Part model, mm, in its own coordinate system. A direction names the side the tool comes from. Give positions to 0.01 mm unless a question says otherwise; leave off trailing zeros. Write each loop counter-clockwise with the first axis right and the second up, starting at its lowest first coordinate (ties: lowest second). Pieces come first, ordered by that corner, then holes. Notation, with made-up numbers: M 58,78.5 L 109,78.5 A28 ccw 109,116.5 Z; hole C 85.25,57.5 d10. An arc over 180 degrees is marked long. Use a Markdown table: item, result.
```python
from build123d import *

# Parameters (mm, degrees)
SKETCH1_R           = 20
BOSS_EXTRUDE1_DEPTH = 6
SKETCH2_R           = 2
SKETCH2_R_2         = 1.5
CUT_EXTRUDE1_DEPTH  = 6
SKETCH4_R           = 3
CUT_EXTRUDE2_DEPTH  = 3.1


with BuildPart() as part:
    # Sketch1 → Boss-Extrude1 (new body)
    with BuildSketch(Plane.XY):
        Circle(SKETCH1_R)
    extrude(amount=BOSS_EXTRUDE1_DEPTH)

    # Sketch2 → Cut-Extrude1 (cut)
    with BuildSketch(Plane(origin=(0, 0, 0), x_dir=(-1, 0, 0), z_dir=(0, 0, -1))):
        with Locations((0, 16)):
            Circle(SKETCH2_R)
        with Locations((11.313708499, 11.313708499)):
            Circle(SKETCH2_R)
        with Locations((16, 0)):
            Circle(SKETCH2_R)
        with Locations((11.313708499, -11.313708499)):
            Circle(SKETCH2_R)
        with Locations((0, -16)):
            Circle(SKETCH2_R)
        with Locations((-11.313708499, -11.313708499)):
            Circle(SKETCH2_R)
        with Locations((-16, 0)):
            Circle(SKETCH2_R)
        with Locations((-11.313708499, 11.313708499)):
            Circle(SKETCH2_R)
        with Locations((-4.949747468, -4.949747468)):
            Circle(SKETCH2_R_2)
        with Locations((-4.949747468, 4.949747468)):
            Circle(SKETCH2_R_2)
        with Locations((4.949747468, 4.949747468)):
            Circle(SKETCH2_R_2)
        with Locations((4.949747468, -4.949747468)):
            Circle(SKETCH2_R_2)
    extrude(amount=-CUT_EXTRUDE1_DEPTH, mode=Mode.SUBTRACT)

    # Sketch4 → Cut-Extrude2 (cut)
    with BuildSketch(Plane(origin=(0, 0, 0), x_dir=(-1, 0, 0), z_dir=(0, 0, -1))):
        with Locations((-4.949747468, 4.949747468)):
            Circle(SKETCH4_R)
        with Locations((4.949747468, 4.949747468)):
            Circle(SKETCH4_R)
        with Locations((4.949747468, -4.949747468)):
            Circle(SKETCH4_R)
        with Locations((-4.949747468, -4.949747468)):
            Circle(SKETCH4_R)
    extrude(amount=-CUT_EXTRUDE2_DEPTH, mode=Mode.SUBTRACT)


solid = part.part
```
1. Drop flat-ended pins along their axis: P1, Ø4, axis at x = 4.95, y = 4.95, coming from the -Z side; P2, Ø2, axis at y = -5.5, z = 4, coming from the -X side; P3, Ø2.5, axis at x = -4.95, y = -4.95, coming from the -Z side (3 decimals). Give the stop position or say it passes through.
Findings below:
| item | result |
|---|---|
| P1 | z = 3.1 |
| P2 | x = -19.49 |
| P3 | through |
2. Cut at A-A, the plane y = 0. Give the cut face in (x, z), then the cut area to 3 significant figures.
Findings below:
| item | result |
|---|---|
| outline | M -20,0 L -18,0 L -18,6 L -20,6 Z; M -14,0 L 14,0 L 14,6 L -14,6 Z; M 18,0 L 20,0 L 20,6 L 18,6 Z |
| area | 192 mm2 |
3. Drill centre lines: L1, parallel to Y at x = 0, z = 3.35; L2, parallel to Y at x = 5, z = 2.6; L3, parallel to X at y = -4.5, z = 0.3. Where is each one in solid material? Low to high.
Findings below:
| item | result |
|---|---|
| L1 | -20 to -18, -14 to 14, 18 to 20 |
| L2 | -19.36 to -7.95, -1.95 to 1.95, 7.95 to 19.36 |
| L3 | -19.49 to -7.92, -1.98 to 1.98, 7.92 to 19.49 |
4. Tool access for faces 4 (the cylindrical face through (11.75, 9.36, 2.96)), 5 (the flat face through (-6.2, 3.7, 3.1)): list every direction of +Z, -Z, +X, -X, +Y, -Y with a clear straight run to the whole face (end or side of a thin tool).
Findings below:
| item | result |
|---|---|
| face 4 | +Z, -Z |
| face 5 | -Z |
5. Two-plate mould, pull along Y, no slides. Class faces 1 (the cylindrical face through (-4.336, -19.524, 2.958)), 2 (the flat face through (0, 0, 6)), 3 (the cylindrical face through (-14.4, -1.2, 3)): released by +Y, released by -Y, zero draft, split by the parting line, or undercut.
Findings below:
| item | result |
|---|---|
| face 1 | split by the parting line |
| face 2 | zero draft |
| face 3 | undercut |
6. Cut at B-B, the plane x = 16. Give the cut face in (y, z), then the cut area to 3 significant figures.
Findings below:
| item | result |
|---|---|
| outline | M -12,0 L -2,0 L -2,6 L -12,6 Z; M 2,0 L 12,0 L 12,6 L 2,6 Z |
| area | 120 mm2 |
